Here's how the part is built. I have some questions about the finished solid (model axes, mm). Face numbers are marked on the shaded views. A direction names the side the tool comes from. Coordinates: 2 decimals unless noted, no trailing zeros. Order: outer loops, then holes, each group sorted by start corner. A loop starts at its lowest first (then second) coordinate and runs counter-clockwise, first axis right, second up.
```python
from build123d import *

# Parameters (mm, degrees)
SKETCH_1_W      = 36
SKETCH_1_H      = 37
EXTRUDE_1_DEPTH = 6
SKETCH_2_W      = 10
SKETCH_2_H      = 37
EXTRUDE_2_DEPTH = 76
SKETCH_3_W      = 36
SKETCH_3_H      = 37
EXTRUDE_3_DEPTH = 6


with BuildPart() as part:
    # 草图1 → 凸台-拉伸1 (new body)
    with BuildSketch(Plane(origin=(0, 0, 0), x_dir=(1, 0, 0), z_dir=(0, 1, 0))):
        Rectangle(SKETCH_1_W, SKETCH_1_H)
    extrude(amount=EXTRUDE_1_DEPTH)

    # 草图2 → 凸台-拉伸2 (add)
    with BuildSketch(Plane(origin=(0, 6, 0), x_dir=(1, 0, 0), z_dir=(0, 1, 0))):
        Rectangle(SKETCH_2_W, SKETCH_2_H)
    extrude(amount=EXTRUDE_2_DEPTH)

    # 草图3 → 凸台-拉伸3 (add)
    with BuildSketch(Plane(origin=(0, 82, 0), x_dir=(1, 0, 0), z_dir=(0, 1, 0))):
        Rectangle(SKETCH_3_W, SKETCH_3_H)
    extrude(amount=EXTRUDE_3_DEPTH)


solid = part.part
```
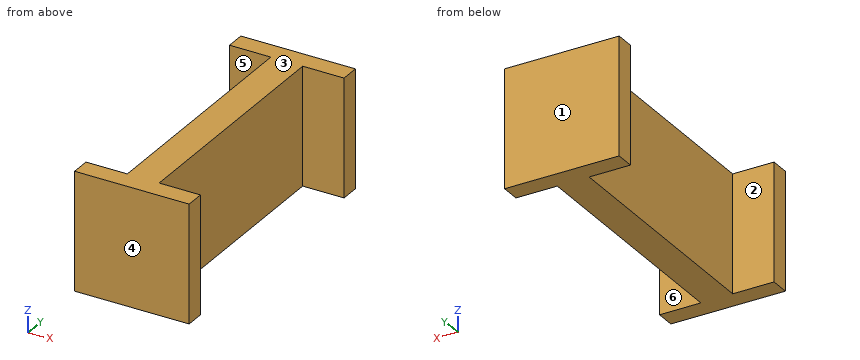
Q1. We'd pull the mould along Y, two halves only. Please class the marked faces 1, 2 and 3: pulls with the +Y half, pulls with the -Y half, needs draft (parallel to the pull), parting line crosses it, or undercut.
Q2. I need wall thicknesses on L1, parallel to Y at x = 14.5, z = -3; L2, parallel to X at y = 75.5, z = 13. Which ranges of each line are inside material? Lowest first, please.
Q3. If we section it at A-A on x = -16: Write out the boundary of the cut face in (y, z), then the cut area to 3 significant figures.
Q4. For the marked faces 4, 5 and 6, which set-ups out of +Z, -Z, +X, -X, +Y, -Y let a thin tool reach every point of the face, with its end or its side?
Q5. Will these pins go through, and if not, where does the flat tip stop? pin 1 (18.5 mm diameter, centred on y = 47, z = 7.5, fed in from +X); pin 2 (11 mm diameter, centred on y = 33.5, z = -2, fed in from -X).
Q6. If we section it at C-C on y = 41: Write out the boundary of the cut face in (x, z), then the cut area to 3 significant figures.
Q7. If we section it at B-B on z = -13: Write out the boundary of the cut face in (x, y).
Reply:
1. face 1: pulls with the +Y half
1. face 2: undercut
1. face 3: needs draft
2. L1: y = 0 to 6, 82 to 88
2. L2: x = -5 to 5
3. outline: (0, -18.5) - (6, -18.5) - (6, 18.5) - (0, 18.5) - close; (82, -18.5) - (88, -18.5) - (88, 18.5) - (82, 18.5) - close
3. area: 444 mm2
4. face 4: +Z, -Z, +X, -X, -Y
4. face 5: +Z, -Z, -X
4. face 6: +Z, -Z, +X
5. pin 1: stops at x = 5
5. pin 2: stops at x = -5
6. outline: (-5, -18.5) - (5, -18.5) - (5, 18.5) - (-5, 18.5) - close
6. area: 370 mm2
7. outline: (-18, 0) - (18, 0) - (18, 6) - (5, 6) - (5, 82) - (18, 82) - (18, 88) - (-18, 88) - (-18, 82) - (-5, 82) - (-5, 6) - (-18, 6) - close
